```python
from build123d import *

# Parameters (mm, degrees)
SKETCH1_W                       = 20.32
SKETCH1_H                       = 3.175
BOSS_EXTRUDE2_DEPTH             = 4.445
SKETCH3_R                       = 2.54
BOSS_EXTRUDE3_DEPTH             = 1.905
SKETCH4_W                       = 17.78
SKETCH4_H                       = 5.08
CUT_EXTRUDE1_DEPTH              = 1.905
SKETCH5_R                       = 1.905
CUT_EXTRUDE2_DEPTH              = 2.54
SKETCH6_R                       = 1.905
SKETCH6_R_2                     = 0.9525
BOSS_EXTRUDE4_DEPTH             = 1.905
BOSS_EXTRUDE5_DEPTH             = 1.27
BOSS_EXTRUDE6_REACH             = 6.445
SKETCH9_R                       = 1.27
BOSS_EXTRUDE6_DIRECTION_2_REACH = 6.445


with BuildPart() as part:
    # Sketch1 → Boss-Extrude2 (new body, symmetric)
    with BuildSketch(Plane.XY):
        with Locations((0, -1.5875)):
            Rectangle(SKETCH1_W, SKETCH1_H)
    extrude(amount=BOSS_EXTRUDE2_DEPTH, both=True)

    # Sketch3 → Boss-Extrude3 (add)
    with BuildSketch(Plane(origin=(0, 0, 0), x_dir=(1, 0, 0), z_dir=(0, 1, 0))):
        with Locations((-5.08, 0)):
            Circle(SKETCH3_R)
        with Locations((5.08, 0)):
            Circle(SKETCH3_R)
    extrude(amount=BOSS_EXTRUDE3_DEPTH)

    # Sketch4 → Cut-Extrude1 (cut)
    with BuildSketch(Plane.XZ.offset(3.175)):
        Rectangle(SKETCH4_W, SKETCH4_H)
    extrude(amount=-CUT_EXTRUDE1_DEPTH, mode=Mode.SUBTRACT)

    # Sketch5 → Cut-Extrude2 (cut)
    with BuildSketch(Plane.XZ.offset(1.27)):
        with Locations((-5.08, 0)):
            Circle(SKETCH5_R)
        with Locations((5.08, 0)):
            Circle(SKETCH5_R)
    extrude(amount=-CUT_EXTRUDE2_DEPTH, mode=Mode.SUBTRACT)

    # Sketch6 → Boss-Extrude4 (add)
    with BuildSketch(Plane.XZ.offset(1.27)):
        Circle(SKETCH6_R)
        Circle(SKETCH6_R_2, mode=Mode.SUBTRACT)
    extrude(amount=BOSS_EXTRUDE4_DEPTH)

    # Sketch8 → Boss-Extrude5 (add)
    with BuildSketch(Plane.XY.offset(4.445)):
        with BuildLine():
            Line((10.16, -3.175), (15.24, -3.175))
            ThreePointArc((15.24, -3.175), (17.248046314, 0.920425987), (12.780655575, 0))
            Line((12.780655575, 0), (10.16, 0))
            Line((10.16, 0), (10.16, -3.175))
        make_face()
    boss_extrude5 = extrude(amount=-BOSS_EXTRUDE5_DEPTH)

    # Mirror1: Boss-Extrude5 across plane
    add(boss_extrude5.mirror(Plane.XY))

    # Sketch9 → Boss-Extrude6 (add, up to next)
    with BuildSketch(Plane.XY, mode=Mode.PRIVATE) as boss_extrude6_sk1:
        with Locations((15.24, -0.635)):
            Circle(SKETCH9_R)
    boss_extrude6_tool1 = extrude(boss_extrude6_sk1.sketch, amount=BOSS_EXTRUDE6_REACH, mode=Mode.PRIVATE) - part.part
    add(boss_extrude6_tool1.solids().sort_by_distance((15.24, -0.635, 0))[0])

    # Sketch9 → Boss-Extrude6 direction 2 (add, up to next)
    with BuildSketch(Plane.XY, mode=Mode.PRIVATE) as boss_extrude6_direction_2_sk1:
        with Locations((15.24, -0.635)):
            Circle(SKETCH9_R)
    boss_extrude6_direction_2_tool1 = extrude(boss_extrude6_direction_2_sk1.sketch, amount=-BOSS_EXTRUDE6_DIRECTION_2_REACH, mode=Mode.PRIVATE) - part.part
    add(boss_extrude6_direction_2_tool1.solids().sort_by_distance((15.24, -0.635, 0))[0])


solid = part.part
```
CAD build for the part. Positions are in the model's coordinates, mm. A direction names the side the tool comes from. Round coordinates to 2 decimals unless told otherwise and drop trailing zeros. Order: outer loops, then holes, each group sorted by start corner. A loop starts at its lowest first (then second) coordinate and runs counter-clockwise, first axis right, second up. Notation, with made-up numbers: (69.25, -15) - (94.25, -15) arc R14 ccw to (94.25, -3) - close; hole circle Ø11 at (0.25, 65.5). An arc over 180 degrees is marked (long way). Answer as CSV lines item,"result". Start each with the question number.
1. Pull direction X, two halves, no side cores. Call faces 4 (the face through (-7.096, 0.939, 1.546)), 5 (the face through (0, -3.175, -3)), 6 (the face through (0, -2, 2.54)), 7 (the face through (17.296, 0.857, 3.819)): +X half, -X half, draft (parallel to the pull), parting line (faces both ways), or undercut.
2. Saw through at D-D, the plane x = 5.08. Write the cut outline in (y, z) (3 decimals), and give its area (3 significant figures).
3. Pin check, flat tips, straight feed: pin 1 (4 mm diameter, centred on x = 5, z = 0, fed in from -Y); pin 2 (1 mm diameter, centred on y = 1, z = 3.5, fed in from +X); pin 3 (1 mm diameter, centred on y = -2.5, z = 0.5, fed in from +X). Stop position of each tip, or through.
4. Saw through at B-B, the plane y = -2.15. Write the cut outline in (x, z) (1 decimal), and give its area (3 significant figures).
5. Saw through at A-A, the plane x = 11.5. Write the cut outline in (y, z) (3 decimals).
6. Tool access for faces 1 (the face through (13.9, -1.2, 3.175)), 2 (the face through (-2.1, -1.27, 0)), 3 (the face through (2.542, 0.939, -0.112)): list every direction of +Z, -Z, +X, -X, +Y, -Y with a clear straight run to the whole face (end or side of a thin tool).
7. Drill centre lines: L1, parallel to Z at x = 0, y = -2.05 (1 decimal); L2, parallel to Z at x = -7.5, y = -2.05 (3 decimals); L3, parallel to Z at x = -1.5, y = -2.45 (3 decimals). Where is each one in solid material? Low to high. Write a range as [from, to].
Model answer:
1,face 4,"undercut"
1,face 5,"draft"
1,face 6,"undercut"
1,face 7,"parting line"
2,outline,"(-3.175, -4.445) - (0, -4.445) - (0, -2.54) - (1.905, -2.54) - (1.905, 2.54) - (0, 2.54) - (0, 4.445) - (-3.175, 4.445) - (-3.175, 2.54) - (-1.27, 2.54) - (-1.27, 1.905) - (1.27, 1.905) - (1.27, -1.905) - (-1.27, -1.905) - (-1.27, -2.54) - (-3.175, -2.54) - close"
2,area,"18.5 mm²"
3,pin 1,"stops at y = -1.27"
3,pin 2,"stops at x = 17.51"
3,pin 3,"stops at x = 10.16"
4,outline,"(-10.2, -4.4) - (17.3, -4.4) - (17.3, -3.2) - (10.2, -3.2) - (10.2, 3.2) - (17.3, 3.2) - (17.3, 4.4) - (-10.2, 4.4) - close; circle Ø3.8 at (0, 0); hole (-8.9, -2.5) - (8.9, -2.5) - (8.9, 2.5) - (-8.9, 2.5) - close; hole circle Ø1.9 at (0, 0)"
4,area,"117 mm²"
5,outline,"(-3.175, -4.445) - (0, -4.445) - (0, -3.175) - (-3.175, -3.175) - close; (-3.175, 3.175) - (0, 3.175) - (0, 4.445) - (-3.175, 4.445) - close"
6,face 1,"none"
6,face 2,"-Y"
6,face 3,"+Y"
7,L1,"z = [-4.4, -2.5], [-1.9, -1], [1, 1.9], [2.5, 4.4]"
7,L2,"z = [-4.445, -2.54], [2.54, 4.445]"
7,L3,"z = [-4.445, -2.54], [-1.174, 1.174], [2.54, 4.445]"
